The listing builds one solid part. Answer for the finished solid, in the listing's coordinates (mm). A direction names the side the tool comes from. Coordinates: 2 decimals unless noted, no trailing zeros. Order: outer loops, then holes, each group sorted by start corner. A loop starts at its lowest first (then second) coordinate and runs counter-clockwise, first axis right, second up.
from build123d import *

# Parameters (mm, degrees)
FILLET2_R                = 6.35
FILLET3_R                = 6.35
CUT_EXTRUDE1_DEPTH       = 278.154041177
CUT_EXTRUDE1_DEPTH_BACK  = 278.154041177
SKETCH2_R                = 9.525
CUT_EXTRUDE12_DEPTH      = 283.485800584
CUT_EXTRUDE12_DEPTH_BACK = 283.485800584
SKETCH6_R                = 9.525
SKETCH6_3_R              = 12.7
SKETCH6_3_R_2            = 9.525
CUT_EXTRUDE13_DEPTH      = 256.54
CUT_EXTRUDE10_DEPTH      = 291.299888117
CUT_EXTRUDE10_DEPTH_BACK = 291.299888117
SKETCH5_W                = 230.453515198
SKETCH5_H                = 214.151634883


with BuildPart() as part:
    # Sketch1 → Revolve1 (revolve)
    with BuildSketch(Plane.XY):
        Polygon((0, 0), (-31.75, 0), (-31.75, -101.6), (-82.55, -101.6), (-82.55, -57.15), (-114.3, -57.15), (-114.3, -69.85), (-101.6, -69.85), (-101.6, -158.75), (-114.3, -158.75), (-114.3, -171.45), (-82.55, -171.45), (-82.55, -127), (-15.748, -127), (-15.748, -151.638), (15.875, -151.638), (15.875, -38.1), (0, -38.1), align=None)
    revolve(axis=Axis((44.45, 0, 0), (0, -1, 0)))

    # Fillet2
    fillet2_edges = [part.edges().sort_by_distance(p)[0] for p in [
        (203.2, -171.45, 0),
        (203.2, -158.75, 0),
    ]]
    fillet(fillet2_edges, radius=FILLET2_R - 0.0001)  # a hair under: the kernel refuses the full size

    # Fillet3
    fillet3_edges = [part.edges().sort_by_distance(p)[0] for p in [
        (203.2, -69.85, 0),
        (203.2, -57.15, 0),
    ]]
    fillet(fillet3_edges, radius=FILLET3_R - 0.0001)  # a hair under: the kernel refuses the full size

    # Sketch2 → Cut-Extrude1 (cut, two sides: drawn at the far end of the back side and taken through both)
    with BuildSketch(Plane(origin=(0, -101.6, 0), x_dir=(1, 0, 0), z_dir=(0, 1, 0)).offset(-CUT_EXTRUDE1_DEPTH_BACK)):
        with Locations(Location((-36.548636908, -50.11769467, 0), (0, 0, 180))):
            Circle(SKETCH2_R)
        with Locations(Location((-39.452515217, 45.088029899, 0), (0, 0, 180))):
            Circle(SKETCH2_R)
        with Locations(Location((47.353878309, -95.205724569, 0), (0, 0, 180))):
            Circle(SKETCH2_R)
        with Locations(Location((125.448636908, 50.11769467, 0), (0, 0, 180))):
            Circle(SKETCH2_R)
        with Locations(Location((128.352515217, -45.088029899, 0), (0, 0, 180))):
            Circle(SKETCH2_R)
        with Locations(Location((41.546121691, 95.205724569, 0), (0, 0, 180))):
            Circle(SKETCH2_R)
    extrude(amount=CUT_EXTRUDE1_DEPTH + CUT_EXTRUDE1_DEPTH_BACK, mode=Mode.SUBTRACT)

    # Sketch6 → Cut-Extrude12 (cut, two sides: drawn at the far end of the back side and taken through both)
    with BuildSketch(Plane(origin=(44.45, 0, 0), x_dir=(0, 0, -1), z_dir=(1, 0, 0)).offset(-CUT_EXTRUDE12_DEPTH_BACK)):
        with Locations((0, -19.05)):
            Circle(SKETCH6_R)
    extrude(amount=CUT_EXTRUDE12_DEPTH + CUT_EXTRUDE12_DEPTH_BACK, mode=Mode.SUBTRACT)

    # Sketch6<3> → Cut-Extrude13 (cut)
    with BuildSketch(Plane(origin=(44.45, 0, 0), x_dir=(0, 0, -1), z_dir=(1, 0, 0))):
        with Locations(Location((0, -19.05, 0), (0, 0, 180))):
            Circle(SKETCH6_3_R)
        with Locations(Location((0, -19.05, 0), (0, 0, 270))):
            Circle(SKETCH6_3_R_2, mode=Mode.SUBTRACT)
    extrude(amount=CUT_EXTRUDE13_DEPTH, mode=Mode.SUBTRACT)

    # Sketch5 → Cut-Extrude10 (cut, two sides: drawn at the far end of the back side and taken through both)
    with BuildSketch(Plane(origin=(0, -38.1, 0), x_dir=(1, 0, 0), z_dir=(0, 1, 0)).offset(-CUT_EXTRUDE10_DEPTH_BACK)):
        with Locations((159.676757599, -107.075817442)):
            Rectangle(SKETCH5_W, SKETCH5_H)
    extrude(amount=CUT_EXTRUDE10_DEPTH + CUT_EXTRUDE10_DEPTH_BACK, mode=Mode.SUBTRACT)


solid = part.part
(1) Find section A-A on y = -19.05. Determine the outline of the cut face in (x, z) (3 decimals).
(2) Find the intervals of material crossed by probe 1 along Y at (x, z) = (-23, 0) (3 decimals); probe 2 along Z at (x, y) = (44, -18); probe 3 along Y at (x, z) = (-77.5, 81.5), in increasing order.
(3) Given pin 1 Ø1.5 at (x, z) = (28, -62) entering from -Y; pin 2 Ø3 at (x, z) = (18.5, -24.5) entering from +Y; pin 3 Ø3 at (x, y) = (100, -1.5) entering from +Z, each flat-ended and moving along its own axis, determine where each tip first touches the part or whether it passes through.
(4) The mould has two halves that part along Y. Classify faces 1 (the flat face through (24.1, -38.1, -20.4)), 2 (the cylindrical face through (-15.6, -9.6, 1.2)), 3 (the flat face through (44.45, -115, 138)): pulls with the +Y half, pulls with the -Y half, needs draft (parallel to the pull), parting line crosses it, or undercut.
(5) A tool of negligible diameter and unlimited length cuts with its end or side. For faces 4 (the cylindrical face through (-62.173, -114.922, -99.811)), 5 (the cylindrical face through (-48.27, -148.91, -86.79)), 6 (the cylindrical face through (-11.179, -51.511, -52.075)), 7 (the flat face through (44.45, -77, 51)), from which of +Z, -Z, +X, -X, +Y, -Y can it reach the whole face along a straight path? Write none if from no direction.
Resolved:
1. outline: (-31.152, -9.525) arc R76.2 ccw to (119.584, -12.7) - (87.047, -12.7) arc R44.45 cw to (1.033, -9.525) - close; (-31.152, 9.525) - (1.033, 9.525) arc R44.45 cw to (44.45, 44.45) - (44.45, 76.2) arc R76.2 ccw to start
2. probe 1: y = -127 to -28.575, -9.525 to 0
2. probe 2: z = -76.2 to -44.45, 44.45 to 76.2
2. probe 3: y = -171.45 to -158.75, -69.85 to -57.15
3. pin 1: stops at y = -127
3. pin 2: stops at y = -38.1
3. pin 3: stops at z = 0
4. face 1: pulls with the +Y half
4. face 2: undercut
4. face 3: needs draft
5. face 4: none
5. face 5: -Y
5. face 6: +Y
5. face 7: +Z, +X, +Y, -Y
